Answer from the drawing. Dimensions are ordinates in mm from the lowest x, y and z of the part. Give positions to 0.01 mm unless a question says otherwise; leave off trailing zeros. Loops run counter-clockwise (first coordinate to the right, second up) from the corner with the lowest first, then second, coordinate; pieces in that order, holes last.
Item 1: Section B-B, the plane y = 7.5 is taken. Give the vertices of the cut face in (x, z) (1 decimal).
Item 2: Section D-D, the plane y = 3 is taken. Give the vertices of the cut face in (x, z).
Item 3: Section A-A, the plane x = 7.5 is taken. Give the vertices of the cut face in (y, z), and give its area (3 significant figures).
Item 4: Section C-C, the plane z = 2.8 is taken. Give the vertices of the cut face in (x, y) (1 decimal).
Item 5: Each of these flat-tipped pins is pushed along its axis until it touches: pin 1 Ø1.5 at (x, z) = (38.5, 4) entering from -Y; pin 2 Ø1 at (x, z) = (78.5, 5) entering from +Y; pin 3 Ø1.5 at (y, z) = (35, 2) entering from +X. Where does it stop, or does it pass through?
Item 6: Consider line 1 along Y through (x, z) = (7.5, 2); line 2 along X through (y, z) = (2.5, 2.7); line 3 along Y through (x, z) = (28, 3.5) (1 decimal). Determine where each line is inside the solid, lowest interval first.
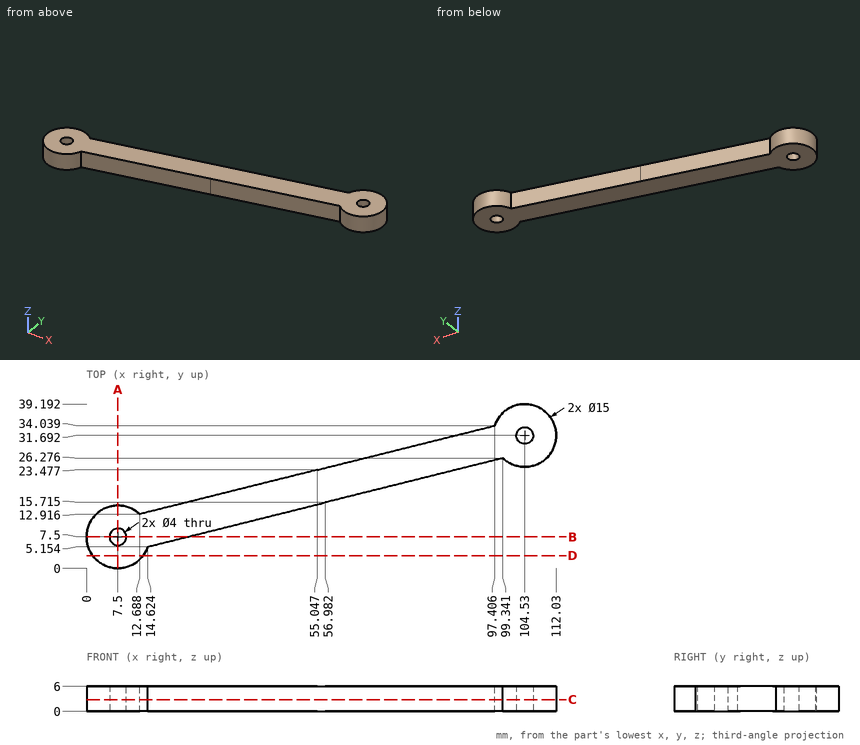
Worked answers:
1. outline: (0, 0) - (5.5, 0) - (5.5, 6) - (0, 6) - close; (9.5, 0) - (24, 0) - (24, 6) - (9.5, 6) - close
2. outline: (1.5, 0) - (13.5, 0) - (13.5, 6) - (1.5, 6) - close
3. outline: (0, 0) - (5.5, 0) - (5.5, 6) - (0, 6) - close; (9.5, 0) - (15, 0) - (15, 6) - (9.5, 6) - close
3. area: 66.0 mm2
4. outline: (12.7, 12.9) arc R7.5 ccw (long way) to (14.6, 5.2) - (99.3, 26.3) arc R7.5 ccw (long way) to (97.4, 34) - close; hole circle Ø4 at (7.5, 7.5); hole circle Ø4 at (104.5, 31.7)
5. pin 1: stops at y = 10.92
5. pin 2: stops at y = 29.45
5. pin 3: stops at x = 111.58
6. line 1: y = 0 to 5.5, 9.5 to 15
6. line 2: x = 1.91 to 13.09
6. line 3: y = 8.5 to 16.7
